```python
from build123d import *

# Parameters (mm, degrees)
MODEL_R                 = 8.05
MODEL_R_2               = 1
MODEL_W                 = 32
MODEL_H                 = 32
MODEL_W_2               = 11.8
MODEL_H_2               = 22.5
SALIENTE_EXTRUIR1_DEPTH = 3
CROQUIS2_W              = 19.999999999
CROQUIS2_H              = 3
SALIENTE_EXTRUIR2_DEPTH = 11
CROQUIS3_R              = 1.5
CORTAR_EXTRUIR1_DEPTH   = 3
REDONDEO1_R             = 2
CROQUIS4_R              = 2.25
CORTAR_EXTRUIR2_DEPTH   = 1
CROQUIS6_R              = 1.5
CORTAR_EXTRUIR4_DEPTH   = 1


with BuildPart() as part:
    # Model → Saliente-Extruir1 (new body)
    with BuildSketch(Plane.XY):
        with BuildLine():
            Line((68.698959582, -55.021016271), (68.698959582, -56.021017288))
            Line((68.698959582, -56.021017288), (48.698959583, -56.021017288))
            Line((48.698959583, -56.021017288), (48.698959583, -55.020994548))
            ThreePointArc((48.698959583, -55.020994548), (48.113181185, -53.606789026), (46.698982323, -53.020994548))
            Line((46.698982323, -53.020994548), (9.698959583, -53.020573857))
            ThreePointArc((9.698959583, -53.020573857), (8.324569809, -52.451282972), (7.755278924, -51.076893199))
            Line((7.755278924, -51.076893199), (7.755278924, -21.120997464))
            ThreePointArc((7.755278924, -21.120997464), (8.341065362, -19.706783901), (9.755278924, -19.120997464))
            Line((9.755278924, -19.120997464), (23.555278924, -19.120997464))
            ThreePointArc((23.555278924, -19.120997464), (24.969492487, -19.706783901), (25.555278924, -21.120997464))
            Line((25.555278924, -21.120997464), (25.555278924, -35.098945331))
            ThreePointArc((25.555278924, -35.098945331), (25.848172143, -35.806052112), (26.555278924, -36.098945331))
            Line((26.555278924, -36.098945331), (27.555278924, -36.098945331))
            ThreePointArc((27.555278924, -36.098945331), (28.262385705, -35.806052112), (28.555278924, -35.098945331))
            Line((28.555278924, -35.098945331), (28.555278924, 17.979002536))
            ThreePointArc((28.555278924, 17.979002536), (31.105578849, 23.945942388), (36.646410135, 27.323454721))
            ThreePointArc((36.646410135, 27.323454721), (36.00468524, 24.677778482), (36.499385848, 22.000712008))
            ThreePointArc((36.499385848, 22.000712008), (41.828182769, 26.639397126), (48.466982875, 29.055966887))
            ThreePointArc((48.466982875, 29.055966887), (47.442986911, 26.551218848), (48.490036744, 24.056020035))
            ThreePointArc((48.490036744, 24.056020035), (53.067544133, 27.431151144), (58.41559095, 29.365958406))
            ThreePointArc((58.41559095, 29.365958406), (60.493005652, 24.667283017), (64.452413363, 21.393708086))
            ThreePointArc((64.452413363, 21.393708086), (71.044296854, 25.835788254), (78.620547187, 28.241081393))
            ThreePointArc((78.620547187, 28.241081393), (80.583592254, 20.972839466), (86.965006165, 16.978037452))
            ThreePointArc((86.965006165, 16.978037452), (88.174666897, 16.217466641), (88.895278924, 14.983584414))
            Line((88.895278924, 14.983584414), (88.895278924, -35.070997464))
            ThreePointArc((88.895278924, -35.070997464), (89.188172143, -35.778104245), (89.895278924, -36.070997464))
            Line((89.895278924, -36.070997464), (90.898959582, -36.070997464))
            ThreePointArc((90.898959582, -36.070997464), (91.606066364, -35.778104245), (91.898959582, -35.070997464))
            Line((91.898959582, -35.070997464), (91.898959582, -21.120997464))
            ThreePointArc((91.898959582, -21.120997464), (92.48474602, -19.706783901), (93.898959582, -19.120997464))
            Line((93.898959582, -19.120997464), (107.698959583, -19.120997464))
            ThreePointArc((107.698959583, -19.120997464), (109.113173145, -19.706783901), (109.698959582, -21.120997464))
            Line((109.698959582, -21.120997464), (109.698959582, -51.020997464))
            ThreePointArc((109.698959582, -51.020997464), (109.113173145, -52.435211026), (107.698959583, -53.020997464))
            Line((107.698959583, -53.020997464), (70.698958566, -53.021016271))
            ThreePointArc((70.698958566, -53.021016271), (69.284745661, -53.606803068), (68.698959582, -55.021016271))
        make_face()
        with Locations((71.698959582, 10.979002536)):
            Circle(MODEL_R, mode=Mode.SUBTRACT)
        with Locations((45.698959583, 10.979002536)):
            Circle(MODEL_R, mode=Mode.SUBTRACT)
        with Locations((100.798959583, -21.720997464)):
            Circle(MODEL_R_2, mode=Mode.SUBTRACT)
        with Locations((100.798959583, -49.020997464)):
            Circle(MODEL_R_2, mode=Mode.SUBTRACT)
        with Locations((16.655278924, -49.020997464)):
            Circle(MODEL_R_2, mode=Mode.SUBTRACT)
        with Locations((16.655278924, -21.720997464)):
            Circle(MODEL_R_2, mode=Mode.SUBTRACT)
        with Locations((58.698959582, -20.020997464)):
            Rectangle(MODEL_W, MODEL_H, mode=Mode.SUBTRACT)
        with Locations((100.798959582, -35.370997464)):
            Rectangle(MODEL_W_2, MODEL_H_2, mode=Mode.SUBTRACT)
        with Locations((16.655278924, -35.370997464)):
            Rectangle(MODEL_W_2, MODEL_H_2, mode=Mode.SUBTRACT)
    extrude(amount=SALIENTE_EXTRUIR1_DEPTH)

    # Croquis2 → Saliente-Extruir2 (add)
    with BuildSketch(Plane.XY.offset(3)):
        with Locations((58.698959583, -54.521017288)):
            Rectangle(CROQUIS2_W, CROQUIS2_H)
    extrude(amount=-SALIENTE_EXTRUIR2_DEPTH)

    # Croquis3 → Cortar-Extruir1 (cut)
    with BuildSketch(Plane(origin=(0, -53.021017288, 0), x_dir=(1, 0, 0), z_dir=(0, 1, 0))):
        with Locations((52.698959583, 3.5)):
            Circle(CROQUIS3_R)
        with Locations((64.698959583, 3.5)):
            Circle(CROQUIS3_R)
    extrude(amount=-CORTAR_EXTRUIR1_DEPTH, mode=Mode.SUBTRACT)

    # Redondeo1
    redondeo1_edges = [part.edges().sort_by_distance(p)[0] for p in [
        (48.698959583, -54.521017288, -8),
        (68.698959582, -54.521017288, -8),
    ]]
    fillet(redondeo1_edges, radius=REDONDEO1_R)

    # Croquis4 → Cortar-Extruir2 (cut)
    with BuildSketch(Plane(origin=(0, -53.021017288, 0), x_dir=(1, 0, 0), z_dir=(0, 1, 0))):
        with Locations((52.698959583, 3.5)):
            Circle(CROQUIS4_R)
        with Locations((64.698959583, 3.5)):
            Circle(CROQUIS4_R)
    extrude(amount=-CORTAR_EXTRUIR2_DEPTH, mode=Mode.SUBTRACT)

    # Croquis6 → Cortar-Extruir4 (cut)
    with BuildSketch(Plane.XY.offset(3)):
        with Locations((16.655278924, -21.720997464)):
            Circle(CROQUIS6_R)
        with Locations((16.655278924, -49.020997464)):
            Circle(CROQUIS6_R)
        with Locations((100.798959583, -49.020997464)):
            Circle(CROQUIS6_R)
        with Locations((100.798959583, -21.720997464)):
            Circle(CROQUIS6_R)
    extrude(amount=-CORTAR_EXTRUIR4_DEPTH, mode=Mode.SUBTRACT)


solid = part.part
```
For this review, take the finished solid that the model builds, in its own axes (mm). A direction names the side the tool comes from. Give positions to 0.01 mm unless a question says otherwise; leave off trailing zeros. Write each loop counter-clockwise with the first axis right and the second up, starting at its lowest first coordinate (ties: lowest second). Pieces come first, ordered by that corner, then holes.
Item 1: Machinability: for faces 1 (the face through (58, -36.021, 1)), 2 (the face through (102.23, -21.27, 2.51)), 3 (the face through (59, -53.021, -4)), which of the approach directions +Z, -Z, +X, -X, +Y, -Y give a long, thin tool a straight path to every point of the face, cutting with its end or side? Answer none if there is none.
Item 2: Take a section at A-A (z = -3.5). Give the boundary of the cut face in (x, y).
Item 3: Wall thickness on probe 1 along X at (y, z) = (-53.75, -3.5); probe 2 along X at (y, z) = (-55.55, -3.5); probe 3 along Z at (x, y) = (77, -32.5): over which ranges is each line inside the solid? List them lowest first.
Item 4: Insertion check: P1, Ø1.5, axis at y = -54.5, z = -1.5, coming from the +X side; P2, Ø4, axis at x = 52.7, z = -3.5, coming from the +Y side; P3, Ø3.5, axis at x = 100.8, y = -49.02, coming from the -Z side. Each pin has a flat end and moves straight along its axis. Give the tip position at first contact, or say it passes through.
Item 5: The part is to be moulded in two halves that separate along Z. For faces 4 (the face through (64, -54.021, -2)), 5 (the face through (54.13, -55.01, -3.95)), 6 (the face through (109.699, -36, 1)), 7 (the face through (59, -41, 3)), say which applies: +Z half, -Z half, draft (parallel to the pull), parting line (faces both ways), or undercut.
Established:
1. face 1: +Z, -Z
1. face 2: +Z
1. face 3: -Z, +X, -X, +Y
2. outline: (48.7, -56.02) - (51.2, -56.02) - (51.2, -54.02) - (50.45, -54.02) - (50.45, -53.02) - (48.7, -53.02) - close; (54.2, -56.02) - (63.2, -56.02) - (63.2, -54.02) - (62.45, -54.02) - (62.45, -53.02) - (54.95, -53.02) - (54.95, -54.02) - (54.2, -54.02) - close; (66.2, -56.02) - (68.7, -56.02) - (68.7, -53.02) - (66.95, -53.02) - (66.95, -54.02) - (66.2, -54.02) - close
3. probe 1: x = 48.7 to 50.45, 54.95 to 62.45, 66.95 to 68.7
3. probe 2: x = 48.7 to 51.2, 54.2 to 63.2, 66.2 to 68.7
3. probe 3: z = 0 to 3
4. P1: stops at x = 68.7
4. P2: stops at y = -54.02
4. P3: stops at z = 0
5. face 4: undercut
5. face 5: undercut
5. face 6: draft
5. face 7: +Z half
